Model file for the job. Use its own axes, mm. Face numbers are marked on the shaded views. Round coordinates to 2 decimals unless told otherwise and drop trailing zeros. Loops run counter-clockwise (first coordinate to the right, second up) from the corner with the lowest first, then second, coordinate; pieces in that order, holes last. Notation, with made-up numbers: (-37.5, 71) - (-28.5, 71) arc R12 cw to (-28.5, 82) - close; hole circle Ø3 at (-36.5, -28.5). An arc over 180 degrees is marked (long way). Answer as a JSON object with one key per item and string values.
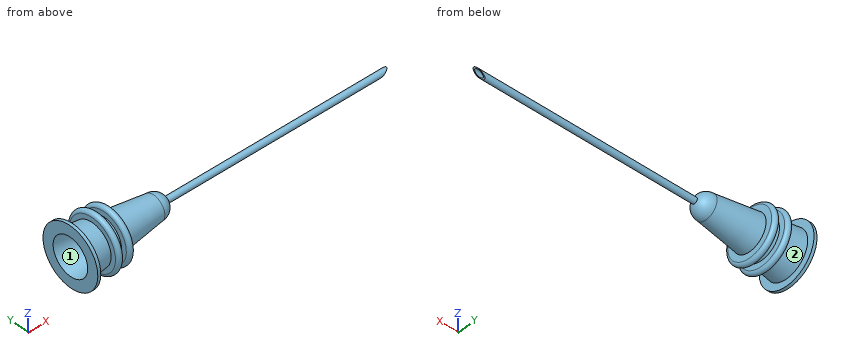
from build123d import *

# Parameters (mm, degrees)
DOME1_FACE_RADIUS       = 2
DOME1_HEIGHT            = 2
SKETCH2_R               = 0.5
CUT_EXTRUDE1_DEPTH      = 15.798648587
SKETCH3_R               = 0.5
SKETCH3_R_2             = 0.375
EXTRUDE_THIN1_DEPTH     = 40
CUT_EXTRUDE2_DEPTH      = 40.635842365
CUT_EXTRUDE2_DEPTH_BACK = 40.635842365
SKETCH4_R               = 3.5
CUT_EXTRUDE4_DEPTH      = 40.635842464
CUT_EXTRUDE4_DEPTH_BACK = 40.635842464
SKETCH5_R               = 5


with BuildPart() as part:
    # Sketch1 → Revolve1 (revolve)
    with BuildSketch(Plane.XY, mode=Mode.PRIVATE) as revolve1_sk:
        with BuildLine():
            Line((0, 0), (0, 2))
            Line((0, 2), (-7.3, 2.99628656))
            Line((-7.3, 2.99628656), (-7.3, 4))
            ThreePointArc((-7.3, 4), (-7.8, 4.5), (-8.3, 4))
            Line((-8.3, 4), (-8.3, 3.132764171))
            Line((-8.3, 3.132764171), (-9.3, 3.269241782))
            Line((-9.3, 3.269241782), (-9.3, 4.2))
            ThreePointArc((-9.3, 4.2), (-9.8, 4.7), (-10.3, 4.2))
            Line((-10.3, 4.2), (-10.3, 3.405719393))
            Line((-10.3, 3.405719393), (-13.5, 3.842447748))
            Line((-13.5, 3.842447748), (-13.5, 5))
            Line((-13.5, 5), (-14, 5))
            Line((-14, 5), (-14, 3.153733977))
            Line((-14, 3.153733977), (-1, 1.379525035))
            Line((-1, 1.379525035), (-1, 0))
            Line((-1, 0), (0, 0))
        make_face()
    revolve(revolve1_sk.sketch.rotate(Axis((0, 0, 0), (-1, 0, 0)), 90), axis=Axis((0, 0, 0), (-1, 0, 0)))

    # Dome1: a dome of height H over a round flat face of radius A is a cap of a sphere of radius (A * A + H * H) / (2 * H)
    dome1_r = (DOME1_FACE_RADIUS * DOME1_FACE_RADIUS + DOME1_HEIGHT * DOME1_HEIGHT) / (2 * DOME1_HEIGHT)
    dome1_base = Plane((0, 0, 0), z_dir=(1, 0, 0))
    with Locations(dome1_base.offset(DOME1_HEIGHT - dome1_r)):
        dome1_ball = Sphere(dome1_r, mode=Mode.PRIVATE)
    add(split(dome1_ball, bisect_by=dome1_base, keep=Keep.TOP, mode=Mode.PRIVATE))

    # Sketch2 → Cut-Extrude1 (cut, through all)
    with BuildSketch(Plane.ZY.offset(1)):
        Circle(SKETCH2_R)
    extrude(amount=-CUT_EXTRUDE1_DEPTH, mode=Mode.SUBTRACT)

    # Sketch3 → Extrude-Thin1 (add)
    with BuildSketch(Plane.ZY.offset(1)):
        Circle(SKETCH3_R)
        Circle(SKETCH3_R_2, mode=Mode.SUBTRACT)
    extrude(amount=-EXTRUDE_THIN1_DEPTH)

    # Sketch4 → Cut-Extrude2 (cut, two sides: drawn at the far end of the back side and taken through both)
    with BuildSketch(Plane(origin=(0, 0, 0), x_dir=(1, 0, 0), z_dir=(0, 1, 0)).offset(-CUT_EXTRUDE2_DEPTH_BACK)):
        with Locations((39, 3.5)):
            Circle(SKETCH4_R)
    extrude(amount=CUT_EXTRUDE2_DEPTH + CUT_EXTRUDE2_DEPTH_BACK, mode=Mode.SUBTRACT)

    # Sketch5 → Cut-Extrude4 (cut, two sides: drawn at the far end of the back side and taken through both)
    with BuildSketch(Plane(origin=(0, 0, 0), x_dir=(1, 0, 0), z_dir=(0, 1, 0)).offset(-CUT_EXTRUDE4_DEPTH_BACK)):
        with Locations((41, 4.082575695)):
            Circle(SKETCH5_R)
    extrude(amount=CUT_EXTRUDE4_DEPTH + CUT_EXTRUDE4_DEPTH_BACK, mode=Mode.SUBTRACT)


solid = part.part
1) Two-plate mould, pull along Z, no slides. Class the marked faces 1 and 2: pulls with the +Z half, pulls with the -Z half, needs draft (parallel to the pull), parting line crosses it, or undercut.
Values follow:
{"face 1": "undercut", "face 2": "parting line crosses it"}
2) Drop flat-ended pins along their axis: P1, Ø4, axis at y = -4, z = 3.5, coming from the +X side; P2, Ø1, axis at x = 15, y = 2, coming from the -Z side; P3, Ø6, axis at x = -1.5, y = 0.5, coming from the -Z side; P4, Ø1.5, axis at x = -8, y = 2.5, coming from the +Z side. Give the stop position or say it passes through.
Values follow:
{"P1": "x = -7.3", "P2": "through", "P3": "z = -2.61", "P4": "z = 4.14"}
3) Probe probe 1 along X at (y, z) = (2.25, 3.25); probe 2 along Y at (x, z) = (-4, -1.25); probe 3 along Z at (x, y) = (-5, 1.5). List the from-to ranges inside material, lowest first.
Values follow:
{"probe 1": "-14 to -13.5, -10.3 to -9.3, -8.3 to -7.3", "probe 2": "-2.22 to -1.28, 1.28 to 2.22", "probe 3": "-2.22 to -1.21, 1.21 to 2.22"}
4) Slice it at A-A on x = 15. List the corners of the cut face in (y, z) (3 decimals).
Values follow:
{"outline": "circle Ø1 at (0, 0); hole circle Ø0.75 at (0, 0)"}
5) Slice it at B-B on x = -3.5. List the corners of the cut face in (y, z), then the cut area to 3 significant figures.
Values follow:
{"outline": "circle Ø4.96 at (0, 0); hole circle Ø3.44 at (0, 0)", "area": "9.98 mm²"}
